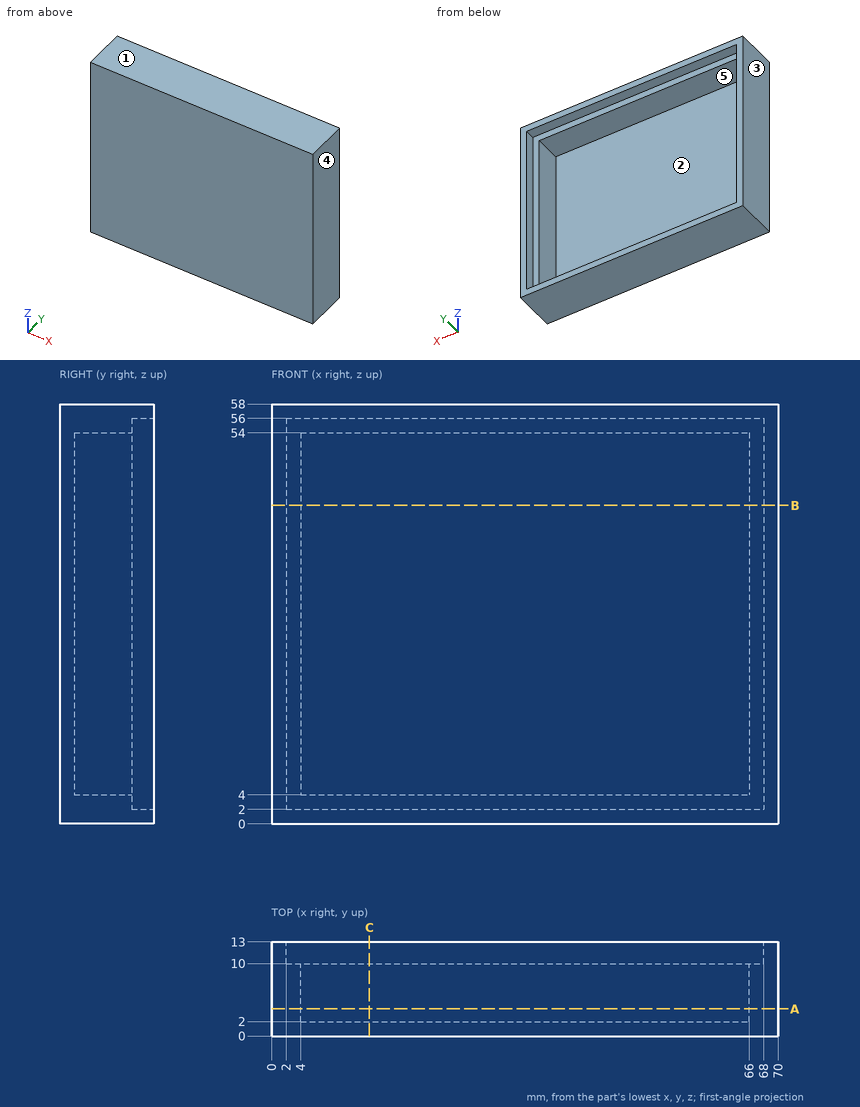
Drawing for the job (mm, zero at the part's lowest x, y, z). A direction names the side the tool comes from. Give positions to 0.01 mm unless a question says otherwise; leave off trailing zeros. Loops run counter-clockwise (first coordinate to the right, second up) from the corner with the lowest first, then second, coordinate; pieces in that order, holes last. Notation, with made-up numbers: M -19,4.25 L 4,4.25 A32 cw 4,33.25 Z; hole C -6.75,57 d11. An arc over 180 degrees is marked long. Use one line per item in the form item = value.
Item 1: Slice it at A-A (y = 3.75). List the corners of the cut face in (x, z).
Determined:
outline = M 0,0 L 70,0 L 70,58 L 0,58 Z; hole M 4,4 L 66,4 L 66,54 L 4,54 Z
Item 2: Which spindle directions (+Z, -Z, +X, -X, +Y, -Y) get a long thin tool onto all of the face, cutting with end or side? Do the marked faces 4 and 5. Say none if no direction does.
Determined:
face_4 = +Z, -Z, +X, +Y, -Y
face_5 = +Y
Item 3: Drill centre lines: probe 1 along X at (y, z) = (8, 44); probe 2 along Z at (x, y) = (33.5, 3); probe 3 along X at (y, z) = (12, 10). Where is each one in solid material? Low to high. Write a range as from..to.
Determined:
probe_1 = 0..4, 66..70
probe_2 = 0..4, 54..58
probe_3 = 0..2, 68..70
Item 4: Flat gauge pin, fed straight in: pin 1 (6 mm diameter, centred on x = 19.5, z = 22, fed in from +Y). Where does the tip first touch, or does it go through?
Determined:
pin_1 = 2
Item 5: Slice it at B-B (z = 44). List the corners of the cut face in (x, y).
Determined:
outline = M 0,0 L 70,0 L 70,13 L 68,13 L 68,10 L 66,10 L 66,2 L 4,2 L 4,10 L 2,10 L 2,13 L 0,13 Z
Item 6: Slice it at C-C (x = 13.5). List the corners of the cut face in (y, z), plus the area to 3 significant figures.
Determined:
outline = M 0,0 L 13,0 L 13,2 L 10,2 L 10,4 L 2,4 L 2,54 L 10,54 L 10,56 L 13,56 L 13,58 L 0,58 Z
area = 192 mm2
Item 7: Two-plate mould, pull along Z, no slides. Class the marked faces 1, 2 and 3: pulls with the +Z half, pulls with the -Z half, needs draft (parallel to the pull), parting line crosses it, or undercut.
Determined:
face_1 = pulls with the +Z half
face_2 = undercut
face_3 = needs draft
